from build123d import *

# Parameters (mm, degrees)
SKETCH1_W               = 25
SKETCH1_H               = 6.15
CHAMFER1_SIZE           = 0.5
CUT_EXTRUDE1_DEPTH      = 27.469699658
CUT_EXTRUDE1_DEPTH_BACK = 27.469699658
SKETCH3_R               = 2
CUT_EXTRUDE3_DEPTH      = 27.469699799
CUT_EXTRUDE3_DEPTH_BACK = 27.469699799
SKETCH6_W               = 11.5
SKETCH6_H               = 3.2
CUT_EXTRUDE4_DEPTH      = 27.469699799
CUT_EXTRUDE4_DEPTH_BACK = 27.469699799
SKETCH11_R              = 2.15


with BuildPart() as part:
    # Sketch1 → Revolve1 (revolve)
    with BuildSketch(Plane.XY):
        with Locations((12.5, 3.075)):
            Rectangle(SKETCH1_W, SKETCH1_H)
    revolve(axis=Axis((25, 0, 0), (-1, 0, 0)))

    # Chamfer1
    chamfer1_edges = [part.edges().sort_by_distance(p)[0] for p in [
        (0, -6.15, 0),
    ]]
    chamfer(chamfer1_edges, length=CHAMFER1_SIZE)

    # Sketch3 → Cut-Extrude1 (cut, two sides: drawn at the far end of the back side and taken through both)
    with BuildSketch(Plane(origin=(0, 0, 0), x_dir=(1, 0, 0), z_dir=(0, 1, 0)).offset(-CUT_EXTRUDE1_DEPTH_BACK)):
        with Locations((6.7, 0)):
            Circle(SKETCH3_R)
    extrude(amount=CUT_EXTRUDE1_DEPTH + CUT_EXTRUDE1_DEPTH_BACK, mode=Mode.SUBTRACT)

    # Sketch6 → Cut-Extrude3 (cut, two sides: drawn at the far end of the back side and taken through both)
    with BuildSketch(Plane(origin=(0, 0, 0), x_dir=(1, 0, 0), z_dir=(0, 1, 0)).offset(-CUT_EXTRUDE3_DEPTH_BACK)):
        with Locations((19.25, -4.55)):
            Rectangle(SKETCH6_W, SKETCH6_H)
        with Locations((19.25, 4.55)):
            Rectangle(SKETCH6_W, SKETCH6_H)
    extrude(amount=CUT_EXTRUDE3_DEPTH + CUT_EXTRUDE3_DEPTH_BACK, mode=Mode.SUBTRACT)

    # Sketch11 → Cut-Extrude4 (cut, two sides: drawn at the far end of the back side and taken through both)
    with BuildSketch(Plane.XY.offset(-CUT_EXTRUDE4_DEPTH_BACK)):
        with Locations((20.85, 0)):
            Circle(SKETCH11_R)
    extrude(amount=CUT_EXTRUDE4_DEPTH + CUT_EXTRUDE4_DEPTH_BACK, mode=Mode.SUBTRACT)


solid = part.part
Verification items for the finished model (mm, model axes). A direction names the side the tool comes from. Coordinates: 2 decimals unless noted, no trailing zeros. Order: outer loops, then holes, each group sorted by start corner. A loop starts at its lowest first (then second) coordinate and runs counter-clockwise, first axis right, second up. Notation, with made-up numbers: M 84,-13 L 128,-13 A8 cw 128,-7 Z; hole C 8,16.5 d6. An arc over 180 degrees is marked long. One line per item, written item: value. Start each with the question number.
Item 1: Mould release check, pull along Z, two halves, no side actions. Record for faces 4 (the cylindrical face through (10.199, 5.866, -1.847)), 5 (the cylindrical face through (6.266, -0.086, 1.952)), 6 (the flat face through (13.5, 0, -4)): released by +Z, released by -Z, zero draft, split by the parting line, or undercut.
Item 2: Sectioned sample at B-B (y = 0). Enter the section's corners in (x, z).
Item 3: Sectioned sample at C-C (x = 19). Enter the section's corners in (y, z).
Item 4: Sectioned sample at D-D (x = 15.75). Enter the section's corners in (y, z), then the cut area to 3 significant figures.
Item 5: Scan lines: probe 1 along X at (y, z) = (0, 0); probe 2 along X at (y, z) = (3.75, 0); probe 3 along X at (y, z) = (-3.5, 3.75). Record each from-to range of solid material in increasing order.
Item 6: Access from +Z, -Z, +X, -X, +Y, -Y to the whole of each face (thin tool, end or side, straight path). Record for faces 1 (the flat face through (25, 0, 0)), 2 (the flat face through (13.5, 0, 4)), 3 (the flat face through (18, 0, -2.95)).
Item 7: Sectioned sample at A-A (z = 0). Enter the section's corners in (x, y), then the cut area to 3 significant figures.
Item 8: Gauge pin test, flat ends, axial feed: pin 1 (2 mm diameter, centred on x = 21, z = 3.5, fed in from -Y); pin 2 (1 mm diameter, centred on y = -0.5, z = 4.5, fed in from +X); pin 3 (5.5 mm diameter, centred on x = 20, y = -0.5, fed in from -Z); pin 4 (5 mm diameter, centred on x = 15.5, z = -2.5, fed in from -Y). Record the tip position at first contact, or that the pin passes through.
Conclusion:
1. face 4: split by the parting line
1. face 5: undercut
1. face 6: zero draft
2. outline: M 0,-5.65 L 0.5,-6.15 L 13.5,-6.15 L 13.5,-2.95 L 18.7,-2.95 L 18.7,2.95 L 13.5,2.95 L 13.5,6.15 L 0.5,6.15 L 0,5.65 Z; M 23,-2.95 L 25,-2.95 L 25,2.95 L 23,2.95 Z; hole C 6.7,0 d4
3. outline: M -5.4,-2.95 L -1.1,-2.95 L -1.1,2.95 L -5.4,2.95 A6.15 ccw Z; M 1.1,-2.95 L 5.4,-2.95 A6.15 ccw 5.4,2.95 L 1.1,2.95 Z
4. outline: M -5.4,-2.95 L 5.4,-2.95 A6.15 ccw 5.4,2.95 L -5.4,2.95 A6.15 ccw Z
4. area: 69.7 mm^2
5. probe 1: x = 0 to 4.7, 8.7 to 18.7, 23 to 25
5. probe 2: x = 0 to 4.7, 8.7 to 25
5. probe 3: x = 0 to 13.5
6. face 1: +Z, -Z, +X, +Y, -Y
6. face 2: +Z, +X, +Y, -Y
6. face 3: -Z, +X, +Y, -Y
7. outline: M 0,-5.65 L 0.5,-6.15 L 4.7,-6.15 L 4.7,6.15 L 0.5,6.15 L 0,5.65 Z; M 8.7,-6.15 L 25,-6.15 L 25,6.15 L 8.7,6.15 Z; hole C 20.85,0 d4.3
7. area: 244 mm^2
8. pin 1: stops at y = -5.62
8. pin 2: stops at x = 13.5
8. pin 3: stops at z = -2.95
8. pin 4: stops at y = -6.15
